Build history of the part. All positions in model axes, mm. A direction names the side the tool comes from. Round coordinates to 2 decimals unless told otherwise and drop trailing zeros. Order: outer loops, then holes, each group sorted by start corner. A loop starts at its lowest first (then second) coordinate and runs counter-clockwise, first axis right, second up. Notation, with made-up numbers: (2, -2.5) -> (20, -2.5) arc R9 ccw to (20, 13.5) -> close; hole circle Ø11 at (85.5, -16.75). An arc over 180 degrees is marked (long way). Answer as CSV lines item,"result". Start each with the question number.
```python
from build123d import *

# Parameters (mm, degrees)
SKETCH1_W           = 400
SKETCH1_H           = 400
BOSS_EXTRUDE1_DEPTH = 400
CUT_EXTRUDE1_DEPTH  = 200
CUT_EXTRUDE2_DEPTH  = 10
FILLET1_R           = 10


with BuildPart() as part:
    # Sketch1 → Boss-Extrude1 (new body)
    with BuildSketch(Plane.XY):
        Rectangle(SKETCH1_W, SKETCH1_H)
    extrude(amount=BOSS_EXTRUDE1_DEPTH)

    # Sketch2 → Cut-Extrude1 (cut)
    with BuildSketch(Plane.XY.offset(380)):
        Polygon((160, 200), (-160, 200), (-160, 160), (-200, 160), (-200, -160), (-160, -160), (-160, -200), (160, -200), (160, -160), (200, -160), (200, 160), (160, 160), align=None)
    extrude(amount=-CUT_EXTRUDE1_DEPTH, mode=Mode.SUBTRACT)

    # Sketch3 → Cut-Extrude2 (cut)
    with BuildSketch(Plane.XY.offset(400)):
        Polygon((-150, 0), (-50, 100), (-50, 40), (150, 40), (150, -40), (-50, -40), (-50, -100), align=None)
    extrude(amount=-CUT_EXTRUDE2_DEPTH, mode=Mode.SUBTRACT)

    # Fillet1
    fillet1_edges = [part.edges().sort_by_distance(p)[0] for p in [
        (200, -200, 200),
        (-200, -200, 200),
        (-200, 200, 200),
        (200, 200, 200),
    ]]
    fillet(fillet1_edges, radius=FILLET1_R)


solid = part.part
```
Q1. Two-plate mould, pull along Y, no slides. Class faces 6 (the face through (160, -180, 281)), 7 (the face through (-3, 3, 380)), 8 (the face through (-3, -200, 108)): +Y half, -Y half, draft (parallel to the pull), parting line (faces both ways), or undercut.
Q2. Slice it at A-A, the plane y = -77.5. Write the cut outline in (x, z).
Q3. Probe L1, parallel to Z at x = 75.5, y = -70; L2, parallel to Z at x = -95.5, y = -37.5; L3, parallel to Y at x = 167, z = 228. List the from-to ranges inside material, lowest first.
Q4. Slice it at C-C, the plane x = -109. Write the cut outline in (y, z).
Q5. Slice it at B-B, the plane z = 203. Write the cut outline in (x, y), plus the area to 3 significant figures.
Q6. Slice it at D-D, the plane y = -169. Write the cut outline in (x, z), plus the area to 3 significant figures.
Q7. Which spindle directions (+Z, -Z, +X, -X, +Y, -Y) get a long thin tool onto all of the face, cutting with end or side? Do faces 1 (the face through (-99, -51, 395)), 2 (the face through (-160, 180, 281)), 3 (the face through (-3, 3, 180)), 4 (the face through (-180, 160, 281)), 5 (the face through (-3, 3, 0)). Say none if no direction does.
Solutions:
1,face 6,"draft"
1,face 7,"undercut"
1,face 8,"-Y half"
2,outline,"(-200, 0) -> (200, 0) -> (200, 180) -> (-200, 180) -> close; (-200, 380) -> (200, 380) -> (200, 400) -> (-50, 400) -> (-50, 390) -> (-72.5, 390) -> (-72.5, 400) -> (-200, 400) -> close"
3,L1,"z = 0 to 180, 380 to 400"
3,L2,"z = 0 to 180, 380 to 390"
3,L3,"y = -200 to -160, 160 to 200"
4,outline,"(-200, 0) -> (200, 0) -> (200, 180) -> (-200, 180) -> close; (-200, 380) -> (200, 380) -> (200, 400) -> (41, 400) -> (41, 390) -> (-41, 390) -> (-41, 400) -> (-200, 400) -> close"
5,outline,"(-200, -190) arc R10 ccw to (-190, -200) -> (-160, -200) -> (-160, -160) -> (-200, -160) -> close; (-200, 160) -> (-160, 160) -> (-160, 200) -> (-190, 200) arc R10 ccw to (-200, 190) -> close; (160, -200) -> (190, -200) arc R10 ccw to (200, -190) -> (200, -160) -> (160, -160) -> close; (160, 160) -> (200, 160) -> (200, 190) arc R10 ccw to (190, 200) -> (160, 200) -> close"
5,area,"6,310 mm2"
6,outline,"(-200, 0) -> (200, 0) -> (200, 400) -> (-200, 400) -> close; hole (-160, 180) -> (160, 180) -> (160, 380) -> (-160, 380) -> close"
6,area,"96,000 mm2"
7,face 1,"+Z"
7,face 2,"+Y, -Y"
7,face 3,"none"
7,face 4,"+X, -X"
7,face 5,"-Z, +X, -X, +Y, -Y"
